from build123d import *

# Parameters (mm, degrees)
BOSS_EXTRUDE1_DEPTH                             = 8
SKETCH5_R                                       = 7.5
CUT_EXTRUDE1_DEPTH                              = 192.983723268
CSK_FOR_M5_FLAT_HEAD_MACHINE_SCREW1_D           = 5.5
CSK_FOR_M5_FLAT_HEAD_MACHINE_SCREW1_CSINK_D     = 10.4
CSK_FOR_M5_FLAT_HEAD_MACHINE_SCREW1_CSINK_ANGLE = 90
CUT_EXTRUDE3_DEPTH                              = 192.983723268
CSK_FOR_M5_FLAT_HEAD_MACHINE_SCREW2_D           = 5.5
CSK_FOR_M5_FLAT_HEAD_MACHINE_SCREW2_DEPTH       = 10
CSK_FOR_M5_FLAT_HEAD_MACHINE_SCREW2_CSINK_D     = 10.4
CSK_FOR_M5_FLAT_HEAD_MACHINE_SCREW2_CSINK_ANGLE = 90
CSK_FOR_M5_FLAT_HEAD_MACHINE_SCREW2_TIP         = 1.652366702
CHAMFER1_SIZE                                   = 0.5
CHAMFER3_SIZE                                   = 0.5
CHAMFER4_SIZE                                   = 2
M3X0_5_TAPPED_HOLE1_D                           = 2.5


with BuildPart() as part:
    # Sketch1 → Boss-Extrude1 (new body)
    with BuildSketch(Plane(origin=(0, 0, 0), x_dir=(1, 0, 0), z_dir=(0, 1, 0))):
        Polygon((72.5, 125.573683549), (-72.5, 125.573683549), (-145, 0), (-72.5, -125.573683549), (72.5, -125.573683549), (145, 0), align=None)
    extrude(amount=BOSS_EXTRUDE1_DEPTH)

    # Sketch5 → Cut-Extrude1 (cut, through all)
    with BuildSketch(Plane(origin=(0, 8, 0), x_dir=(1, 0, 0), z_dir=(0, 1, 0))):
        with Locations(Location((0, 0, 0), (0, 0, 270))):
            Circle(SKETCH5_R)
    extrude(amount=-CUT_EXTRUDE1_DEPTH, mode=Mode.SUBTRACT)

    # CSK for M5 Flat Head Machine Screw1 (through all)
    with Locations(Plane(origin=(0, 0, 0), x_dir=(-1, 0, 0), z_dir=(0, -1, 0))):
        with Locations((52.5, 27.5), (17.5, 27.5), (17.5, 72.5), (52.5, 72.5), (-32.565698604, 1.405444566), (-71.536841774, -21.094555434), (-89.036841774, 9.216333699), (-50.065698604, 31.716333699), (15.065698604, -28.905444566), (-2.434301396, -59.216333699), (36.536841774, -81.716333699), (54.036841774, -51.405444566)):
            CounterSinkHole(CSK_FOR_M5_FLAT_HEAD_MACHINE_SCREW1_D / 2, CSK_FOR_M5_FLAT_HEAD_MACHINE_SCREW1_CSINK_D / 2, counter_sink_angle=CSK_FOR_M5_FLAT_HEAD_MACHINE_SCREW1_CSINK_ANGLE)

    # Sketch9 → Cut-Extrude3 (cut, through all)
    with BuildSketch(Plane.XZ):
        with BuildLine():
            Line((26.812177826, -32.440054257), (14.812177826, -11.655444566))
            ThreePointArc((14.812177826, -11.655444566), (16.459292144, -5.508330249), (22.606406461, -7.155444566))
            Line((22.606406461, -7.155444566), (34.606406461, -27.940054257))
            ThreePointArc((34.606406461, -27.940054257), (32.959292144, -34.087168574), (26.812177826, -32.440054257))
        make_face()
        with BuildLine():
            Line((-41.5, -7), (-17.5, -7))
            ThreePointArc((-17.5, -7), (-13, -11.5), (-17.5, -16))
            Line((-17.5, -16), (-41.5, -16))
            ThreePointArc((-41.5, -16), (-46, -11.5), (-41.5, -7))
        make_face()
        with BuildLine():
            Line((14.687822174, 39.440054257), (2.687822174, 18.655444566))
            ThreePointArc((2.687822174, 18.655444566), (-3.459292144, 17.008330249), (-5.106406461, 23.155444566))
            Line((-5.106406461, 23.155444566), (6.893593539, 43.940054257))
            ThreePointArc((6.893593539, 43.940054257), (13.040707856, 45.587168574), (14.687822174, 39.440054257))
        make_face()
    extrude(amount=-CUT_EXTRUDE3_DEPTH, mode=Mode.SUBTRACT)

    # CSK for M5 Flat Head Machine Screw2
    with Locations(Plane(origin=(0, 8, 0), x_dir=(1, 0, 0), z_dir=(0, 1, 0))):
        with Locations((-135, 0), (-67.5, -116.913429511), (67.5, -116.913429511), (135, 0), (67.5, 116.913429511), (-67.5, 116.913429511)):
            CounterSinkHole(CSK_FOR_M5_FLAT_HEAD_MACHINE_SCREW2_D / 2, CSK_FOR_M5_FLAT_HEAD_MACHINE_SCREW2_CSINK_D / 2, depth=CSK_FOR_M5_FLAT_HEAD_MACHINE_SCREW2_DEPTH, counter_sink_angle=CSK_FOR_M5_FLAT_HEAD_MACHINE_SCREW2_CSINK_ANGLE)
            with Locations((0, 0, -(CSK_FOR_M5_FLAT_HEAD_MACHINE_SCREW2_DEPTH + CSK_FOR_M5_FLAT_HEAD_MACHINE_SCREW2_TIP / 2))):  # 118° drill point
                Cone(0, CSK_FOR_M5_FLAT_HEAD_MACHINE_SCREW2_D / 2, CSK_FOR_M5_FLAT_HEAD_MACHINE_SCREW2_TIP, mode=Mode.SUBTRACT)

    # Chamfer1
    chamfer1_edges = [part.edges().sort_by_distance(p)[0] for p in [
        (32.959292144, 8, -34.087168574),
        (20.812177826, 8, -22.047749412),
        (16.459292144, 8, -5.508330249),
        (28.606406461, 8, -17.547749412),
        (32.959292144, 0, -34.087168574),
        (28.606406461, 0, -17.547749412),
        (16.459292144, 0, -5.508330249),
        (20.812177826, 0, -22.047749412),
        (-46, 8, -11.5),
        (-29.5, 8, -7),
        (-13, 8, -11.5),
        (-29.5, 8, -16),
        (-46, 0, -11.5),
        (-29.5, 0, -16),
        (-13, 0, -11.5),
        (-29.5, 0, -7),
        (13.040707856, 8, 45.587168574),
        (8.687822174, 8, 29.047749412),
        (-3.459292144, 8, 17.008330249),
        (0.893593539, 8, 33.547749412),
        (13.040707856, 0, 45.587168574),
        (0.893593539, 0, 33.547749412),
        (-3.459292144, 0, 17.008330249),
        (8.687822174, 0, 29.047749412),
    ]]
    chamfer(chamfer1_edges, length=CHAMFER1_SIZE)

    # Chamfer3
    chamfer3_edges = [part.edges().sort_by_distance(p)[0] for p in [
        (0, 0, -7.5),
        (0, 8, -7.5),
    ]]
    chamfer(chamfer3_edges, length=CHAMFER3_SIZE)

    # Chamfer4
    chamfer4_edges = [part.edges().sort_by_distance(p)[0] for p in [
        (-108.75, 8, -62.786841774),
        (-108.75, 8, 62.786841774),
        (0, 8, 125.573683549),
        (108.75, 8, 62.786841774),
        (108.75, 8, -62.786841774),
        (0, 8, -125.573683549),
    ]]
    chamfer(chamfer4_edges, length=CHAMFER4_SIZE)

    # M3x0.5 Tapped Hole1 (through all)
    with Locations(Plane(origin=(0, 8, 0), x_dir=(1, 0, 0), z_dir=(0, 1, 0))):
        with Locations((97.25, -65.384917986), (105.25, -51.528511525), (8, 116.913429511), (-8, 116.913429511), (-105.25, -51.528511525), (-97.25, -65.384917986)):
            Hole(M3X0_5_TAPPED_HOLE1_D / 2)


solid = part.part
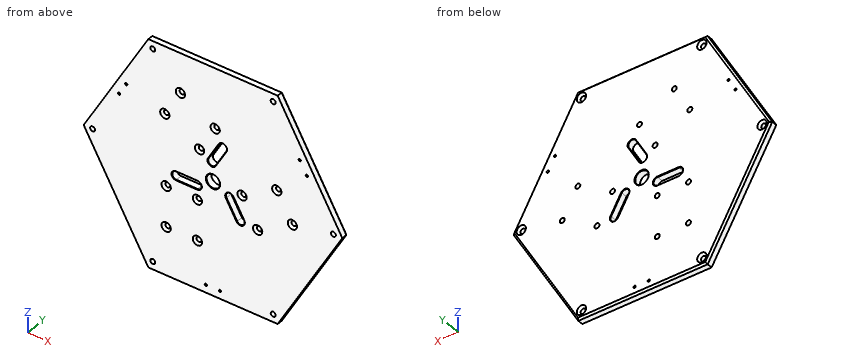
CAD build for the part. Positions are in the model's coordinates, mm. Give positions to 0.01 mm unless a question says otherwise; leave off trailing zeros. Loops run counter-clockwise (first coordinate to the right, second up) from the corner with the lowest first, then second, coordinate; pieces in that order, holes last. Notation, with made-up numbers: M 81.5,82 L 140.5,82 A14 cw 140.5,86 Z; hole C -10,42 d5. An arc over 180 degrees is marked long. Answer in a Markdown table with one row per item. Add a question column.
Item 1: Drop flat-ended pins along their axis: P1, Ø1, axis at y = 4, z = 26, coming from the -X side; P2, Ø9, axis at x = -17.5, z = -72.5, coming from the -Y side; P3, Ø5, axis at x = -67.5, z = -116.91, coming from the +Y side. Give the stop position or say it passes through.
Item 2: Probe probe 1 along Z at (x, y) = (-67.5, 3.6); probe 2 along X at (y, z) = (4, 114.5); probe 3 along X at (y, z) = (3.25, -1). List the from-to ranges inside material, lowest first.
Item 3: Band-saw the part on A-A on x = -111. Give the cut face in (y, z), then the cut area to 3 significant figures.
Reply:
| question | item | result |
|---|---|---|
| 1 | P1 | stops at x = -130.28 |
| 1 | P2 | stops at y = 0.7 |
| 1 | P3 | passes through |
| 2 | probe 1 | z = -125.57 to -119.66, -114.16 to 114.16, 119.66 to 125.57 |
| 2 | probe 2 | x = -78.89 to -68.82, -66.18 to 66.18, 68.82 to 78.89 |
| 2 | probe 3 | x = -144.42 to -137.56, -132.44 to -7.43, 7.43 to 29.85, 35.29 to 132.44, 137.56 to 144.42 |
| 3 | outline | M 0,-58.89 L 6,-58.89 L 8,-54.89 L 8,54.89 L 6,58.89 L 0,58.89 Z |
| 3 | area | 934 mm^2 |
